Check sheet for the modelled part. Datum: model origin and axes. Units: mm. Face numbers are marked on the shaded views. A direction names the side the tool comes from. Round coordinates to 2 decimals unless told otherwise and drop trailing zeros. Loops run counter-clockwise (first coordinate to the right, second up) from the corner with the lowest first, then second, coordinate; pieces in that order, holes last. Notation, with made-up numbers: (-13.75, 73) -> (14.25, 73) arc R19 ccw to (14.25, 80) -> close; hole circle Ø2 at (45.25, 25.5). An arc over 180 degrees is marked (long way). Use one line per item in the form item = value. Start each with the question number.
(1) Go/stop test with flat-tipped pins: pin 1 (6 mm diameter, centred on y = 248, z = 1132, fed in from +X); pin 2 (12.5 mm diameter, centred on x = 37.5, z = 740, fed in from +Y); pin 3 (4 mm diameter, centred on y = 230, z = 1452, fed in from -X). Record where each tip stops, or that it passes through.
(2) Sectioned sample at A-A (y = 256.5). Record the cut outline in (x, z), and give its area (3 significant figures).
(3) Material ranges on probe 1 along Y at (x, z) = (180, 2054); probe 2 along Y at (x, z) = (-15, 2055.25); probe 3 along X at (y, z) = (422, 252.5), recorded low to high. Write a range as [from, to].
(4) Set-up check for the marked faces 3 and 4: record each of +Z, -Z, +X, -X, +Y, -Y from which the full face is reachable in a straight line by a thin tool's end or side.
(5) Draft check along Z on the marked faces 1 and 2. Enter one of: released by +Z, released by -Z, zero draft, split by the parting line, or undercut.
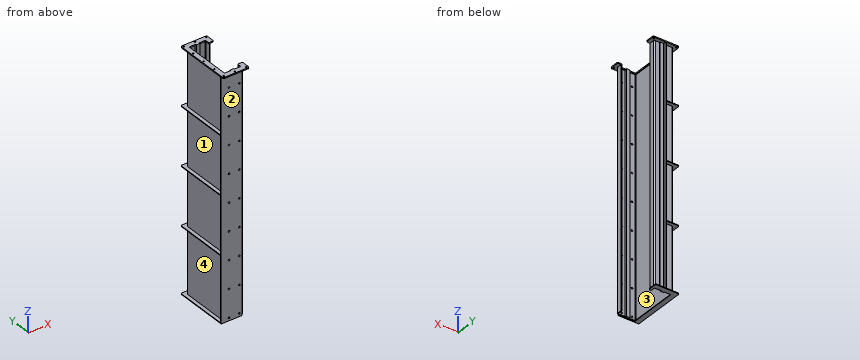
from build123d import *

# Parameters (mm, degrees)
EXTRUDE_1_DEPTH     = 2050
EXTRUDE_2_DEPTH     = 10
SKETCH_3_W          = 40
SKETCH_3_H          = 2050
EXTRUDE_3_DEPTH     = 6
SKETCH_4_W          = 6
SKETCH_4_H          = 2050
EXTRUDE_4_DEPTH     = 24
FILLET_1_R          = 4
FILLET_2_R          = 10
EXTRUDE_5_DEPTH     = 6
EXTRUDE_6_DEPTH     = 6
EXTRUDE_7_DEPTH     = 6
EXTRUDE_8_DEPTH     = 6
SKETCH_9_W          = 180
SKETCH_9_H          = 2056
EXTRUDE_9_DEPTH     = 6
SKETCH_10_W         = 30
SKETCH_10_H         = 14
EXTRUDE_10_DEPTH    = 2066
SKETCH_11_R         = 7
CUT_EXTRUDE_1_DEPTH = 37
SKETCH_13_R         = 6
CUT_EXTRUDE_2_DEPTH = 10


with BuildPart() as part:
    # Sketch 1 → Extrude 1 (new body)
    with BuildSketch(Plane.XY):
        with BuildLine():
            Line((10, 430), (155, 430))
            ThreePointArc((155, 430), (157.828427125, 428.828427125), (159, 426))
            Line((159, 426), (159, 386))
            Line((159, 386), (165, 386))
            Line((165, 386), (165, 426))
            ThreePointArc((165, 426), (162.071067812, 433.071067812), (155, 436))
            Line((155, 436), (10, 436))
            ThreePointArc((10, 436), (2.928932188, 433.071067812), (0, 426))
            Line((0, 426), (0, 10))
            ThreePointArc((0, 10), (2.928932188, 2.928932188), (10, 0))
            Line((10, 0), (155, 0))
            ThreePointArc((155, 0), (162.071067812, 2.928932188), (165, 10))
            Line((165, 10), (165, 50))
            Line((165, 50), (159, 50))
            Line((159, 50), (159, 10))
            ThreePointArc((159, 10), (157.828427125, 7.171572875), (155, 6))
            Line((155, 6), (10, 6))
            ThreePointArc((10, 6), (7.171572875, 7.171572875), (6, 10))
            Line((6, 10), (6, 426))
            ThreePointArc((6, 426), (7.171572875, 428.828427125), (10, 430))
        make_face()
    extrude(amount=EXTRUDE_1_DEPTH)



with BuildPart() as body_2:
    # Sketch 2 → Extrude 2 (new body)
    with BuildSketch(Plane.XY.offset(2050)):
        with BuildLine():
            Line((185, 466), (-20, 466))
            ThreePointArc((-20, 466), (-27.071067812, 463.071067812), (-30, 456))
            Line((-30, 456), (-30, -20))
            ThreePointArc((-30, -20), (-27.071067812, -27.071067812), (-20, -30))
            Line((-20, -30), (185, -30))
            ThreePointArc((185, -30), (192.071067812, -27.071067812), (195, -20))
            Line((195, -20), (195, 40))
            ThreePointArc((195, 40), (192.071067812, 47.071067812), (185, 50))
            Line((185, 50), (157, 50))
            ThreePointArc((157, 50), (154.171572875, 48.828427125), (153, 46))
            Line((153, 46), (153, 16))
            ThreePointArc((153, 16), (151.828427125, 13.171572875), (149, 12))
            Line((149, 12), (16, 12))
            ThreePointArc((16, 12), (13.171572875, 13.171572875), (12, 16))
            Line((12, 16), (12, 420))
            ThreePointArc((12, 420), (13.171572875, 422.828427125), (16, 424))
            Line((16, 424), (149, 424))
            ThreePointArc((149, 424), (151.828427125, 422.828427125), (153, 420))
            Line((153, 420), (153, 390))
            ThreePointArc((153, 390), (154.171572875, 387.171572875), (157, 386))
            Line((157, 386), (185, 386))
            ThreePointArc((185, 386), (192.071067812, 388.928932188), (195, 396))
            Line((195, 396), (195, 456))
            ThreePointArc((195, 456), (192.071067812, 463.071067812), (185, 466))
        make_face()
    extrude(amount=EXTRUDE_2_DEPTH)



with BuildPart() as body_3:
    # Sketch 3 → Extrude 3 (new body)
    with BuildSketch(Plane(origin=(0, 436, 0), x_dir=(1, 0, 0), z_dir=(0, 1, 0))):
        with Locations((100, -1025)):
            Rectangle(SKETCH_3_W, SKETCH_3_H)
    extrude(amount=EXTRUDE_3_DEPTH)


with BuildPart() as body_2_1:
    add(body_2.part)

    add(body_3.part)  # Extrude 4 merges body 3
    # Sketch 4 → Extrude 4 (add)
    with BuildSketch(Plane(origin=(0, 442, 0), x_dir=(1, 0, 0), z_dir=(0, 1, 0))):
        with Locations((83, -1025)):
            Rectangle(SKETCH_4_W, SKETCH_4_H)
    extrude(amount=EXTRUDE_4_DEPTH)

    # Fillet 1
    fillet_1_edges = [body_2_1.edges().sort_by_distance(p)[0] for p in [
        (86, 442, 1025),
    ]]
    fillet(fillet_1_edges, radius=FILLET_1_R)

    # Fillet 2
    fillet_2_edges = [body_2_1.edges().sort_by_distance(p)[0] for p in [
        (80, 436, 1025),
    ]]
    fillet(fillet_2_edges, radius=FILLET_2_R)


with BuildPart() as part_1:
    add(part.part)

    add(body_2_1.part)  # Extrude 5 merges body 2
    # Sketch 5 → Extrude 5 (add)
    with BuildSketch(Plane.XY.offset(1560)):
        with BuildLine():
            Line((0, 0), (-20, 0))
            ThreePointArc((-20, 0), (-27.071067812, 2.928932188), (-30, 10))
            Line((-30, 10), (-30, 456))
            ThreePointArc((-30, 456), (-27.071067812, 463.071067812), (-20, 466))
            Line((-20, 466), (80, 466))
            Line((80, 466), (80, 436))
            Line((80, 436), (10, 436))
            ThreePointArc((10, 436), (2.928932188, 433.071067812), (0, 426))
            Line((0, 426), (0, 0))
        make_face()
    extrude(amount=EXTRUDE_5_DEPTH)

    # Sketch 6 → Extrude 6 (add)
    with BuildSketch(Plane.XY.offset(1060)):
        with BuildLine():
            Line((0, 0), (0, 10))
            Line((0, 10), (0, 426))
            ThreePointArc((0, 426), (2.928932188, 433.071067812), (10, 436))
            Line((10, 436), (80, 436))
            Line((80, 436), (80, 446))
            Line((80, 446), (80, 466))
            Line((80, 466), (-20, 466))
            ThreePointArc((-20, 466), (-27.071067812, 463.071067812), (-30, 456))
            Line((-30, 456), (-30, 10))
            ThreePointArc((-30, 10), (-27.071067812, 2.928932188), (-20, 0))
            Line((-20, 0), (0, 0))
        make_face()
    extrude(amount=EXTRUDE_6_DEPTH)

    # Sketch 7 → Extrude 7 (add)
    with BuildSketch(Plane.XY.offset(560)):
        with BuildLine():
            Line((0, 10), (0, 426))
            ThreePointArc((0, 426), (2.928932188, 433.071067812), (10, 436))
            Line((10, 436), (80, 436))
            Line((80, 436), (80, 446))
            Line((80, 446), (80, 466))
            Line((80, 466), (-20, 466))
            ThreePointArc((-20, 466), (-27.071067812, 463.071067812), (-30, 456))
            Line((-30, 456), (-30, 10))
            ThreePointArc((-30, 10), (-27.071067812, 2.928932188), (-20, 0))
            Line((-20, 0), (0, 0))
            Line((0, 0), (0, 10))
        make_face()
    extrude(amount=EXTRUDE_7_DEPTH)

    # Sketch 8 → Extrude 8 (add)
    with BuildSketch(Plane(origin=(0, 0, 0), x_dir=(-1, 0, 0), z_dir=(0, 0, -1))):
        with BuildLine():
            Line((-12, 0), (30, 0))
            Line((30, 0), (30, 456))
            ThreePointArc((30, 456), (27.071067812, 463.071067812), (20, 466))
            Line((20, 466), (-165, 466))
            ThreePointArc((-165, 466), (-172.071067812, 463.071067812), (-175, 456))
            Line((-175, 456), (-175, 396))
            ThreePointArc((-175, 396), (-172.071067812, 388.928932188), (-165, 386))
            Line((-165, 386), (-157, 386))
            ThreePointArc((-157, 386), (-154.171572875, 387.171572875), (-153, 390))
            Line((-153, 390), (-153, 420))
            ThreePointArc((-153, 420), (-151.828427125, 422.828427125), (-149, 424))
            Line((-149, 424), (-16, 424))
            ThreePointArc((-16, 424), (-13.171572875, 422.828427125), (-12, 420))
            Line((-12, 420), (-12, 0))
        make_face()
    extrude(amount=EXTRUDE_8_DEPTH)

    # Sketch 9 → Extrude 9 (add)
    with BuildSketch(Plane.XZ):
        with Locations((60, 1022)):
            Rectangle(SKETCH_9_W, SKETCH_9_H)
    extrude(amount=EXTRUDE_9_DEPTH)

    # Sketch 10 → Extrude 10 (add)
    with BuildSketch(Plane.XY.offset(2060)):
        with Locations((82.5, 13)):
            Rectangle(SKETCH_10_W, SKETCH_10_H)
        with Locations((82.5, 423)):
            Rectangle(SKETCH_10_W, SKETCH_10_H)
    extrude(amount=-EXTRUDE_10_DEPTH)

    # Sketch 11 → Cut-Extrude 1 (cut, through all)
    with BuildSketch(Plane(origin=(0, 6, 0), x_dir=(1, 0, 0), z_dir=(0, 1, 0))):
        with Locations((37.5, -20)):
            Circle(SKETCH_11_R)
        with Locations((127.5, -20)):
            Circle(SKETCH_11_R)
        with Locations((37.5, -260)):
            Circle(SKETCH_11_R)
        with Locations((127.5, -260)):
            Circle(SKETCH_11_R)
        with Locations((37.5, -500)):
            Circle(SKETCH_11_R)
        with Locations((127.5, -500)):
            Circle(SKETCH_11_R)
        with Locations((37.5, -740)):
            Circle(SKETCH_11_R)
        with Locations((127.5, -740)):
            Circle(SKETCH_11_R)
        with Locations((37.5, -980)):
            Circle(SKETCH_11_R)
        with Locations((127.5, -980)):
            Circle(SKETCH_11_R)
        with Locations((37.5, -1220)):
            Circle(SKETCH_11_R)
        with Locations((127.5, -1220)):
            Circle(SKETCH_11_R)
        with Locations((37.5, -1460)):
            Circle(SKETCH_11_R)
        with Locations((127.5, -1460)):
            Circle(SKETCH_11_R)
        with Locations((37.5, -1700)):
            Circle(SKETCH_11_R)
        with Locations((127.5, -1700)):
            Circle(SKETCH_11_R)
        with Locations((37.5, -1940)):
            Circle(SKETCH_11_R)
        with Locations((127.5, -1940)):
            Circle(SKETCH_11_R)
    extrude(amount=-CUT_EXTRUDE_1_DEPTH, mode=Mode.SUBTRACT)

    # Sketch 13 → Cut-Extrude 2 (cut)
    with BuildSketch(Plane.XY.offset(2060)):
        with Locations((82.5, -15)):
            Circle(SKETCH_13_R)
        with Locations((-15, -15)):
            Circle(SKETCH_13_R)
        with Locations((180, -15)):
            Circle(SKETCH_13_R)
        with Locations((-15, 218)):
            Circle(SKETCH_13_R)
        with Locations((-15, 451)):
            Circle(SKETCH_13_R)
        with Locations((82.5, 451)):
            Circle(SKETCH_13_R)
        with Locations((180, 451)):
            Circle(SKETCH_13_R)
        with Locations((-15, 341)):
            Circle(SKETCH_13_R)
        with Locations((-15, 95)):
            Circle(SKETCH_13_R)
    extrude(amount=-CUT_EXTRUDE_2_DEPTH, mode=Mode.SUBTRACT)


solid = part_1.part
Checks:
q1.pin_1 = 6
q1.pin_2 = 436
q1.pin_3 = 0
q2.outline = (-30, -6) -> (12, -6) -> (12, 0) -> (6, 0) -> (6, 2050) -> (12, 2050) -> (12, 2060) -> (-30, 2060) -> (-30, 2050) -> (0, 2050) -> (0, 1566) -> (-30, 1566) -> (-30, 1560) -> (0, 1560) -> (0, 1066) -> (-30, 1066) -> (-30, 1060) -> (0, 1060) -> (0, 566) -> (-30, 566) -> (-30, 560) -> (0, 560) -> (0, 0) -> (-30, 0) -> close
q2.area = 13,500 mm2
q3.probe_1 = [-30, -21], [-9, 50], [386, 445], [457, 466]
q3.probe_2 = [-30, -21], [-9, 89], [101, 212], [224, 335], [347, 445], [457, 466]
q3.probe_3 = [0, 6], [67.5, 97.5], [159, 165]
q4.face_3 = none
q4.face_4 = -X, +Y
q5.face_1 = undercut
q5.face_2 = zero draft
